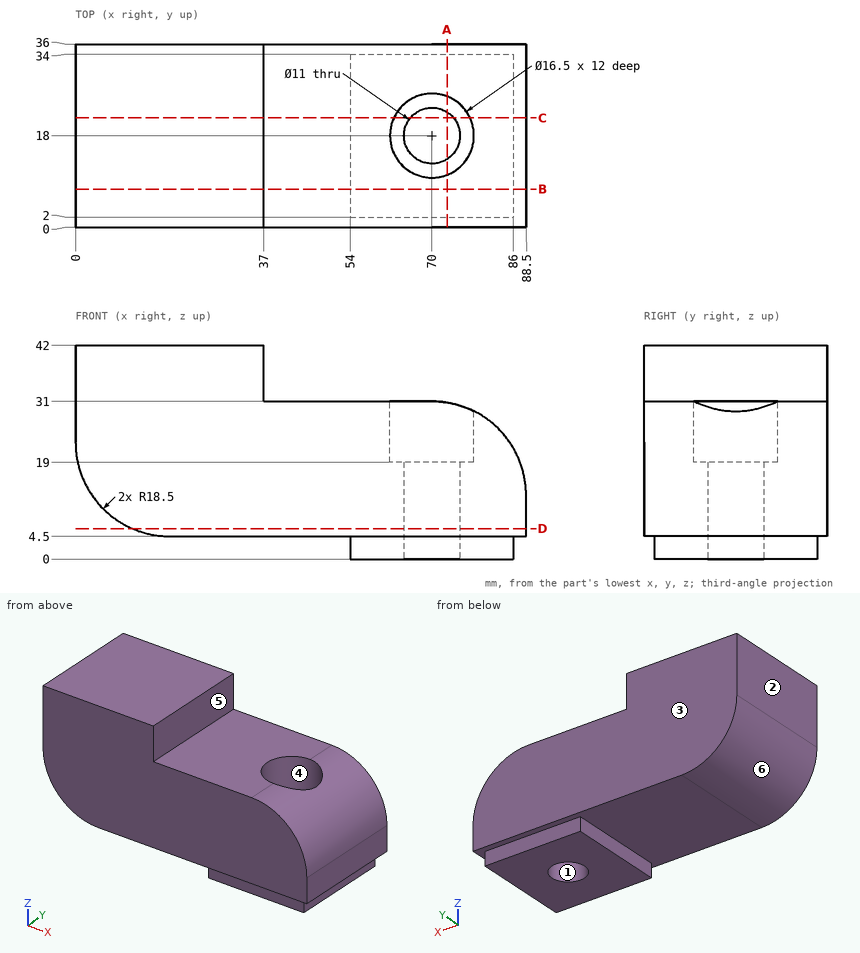
Answer from the drawing. Dimensions are ordinates in mm from the lowest x, y and z of the part. A direction names the side the tool comes from. Round coordinates to 2 decimals unless told otherwise and drop trailing zeros. Write each loop counter-clockwise with the first axis right and the second up, starting at its lowest first coordinate (ties: lowest second). Pieces come first, ordered by that corner, then holes. Notation, with made-up numbers: (59, 41) - (82, 41) arc R27 ccw to (82, 75) - close; hole circle Ø8 at (-3.5, 16). An arc over 180 degrees is marked (long way). One line per item, written item: value.
Q1. Find section A-A (x = 73). Determine the outline of the cut face in (y, z), and give its area (3 significant figures).
The answers:
outline: (0, 4.5) - (2, 4.5) - (2, 0) - (13.39, 0) - (13.39, 19) - (10.31, 19) - (10.31, 30.76) - (0, 30.76) - close; (22.61, 0) - (34, 0) - (34, 4.5) - (36, 4.5) - (36, 30.76) - (25.69, 30.76) - (25.69, 19) - (22.61, 19) - close
area: 733 mm2
Q2. Straight lines are drawn through the part: line 1 (Y direction, x = 70, z = 4); line 2 (Y direction, x = 70, z = 9); line 3 (Z direction, x = 67.5, y = 5.5). For each, find the intervals that lie inside material, in ascending order. Write a range as from..to.
The answers:
line 1: y = 2..12.5, 23.5..34
line 2: y = 0..12.5, 23.5..36
line 3: z = 0..31
Q3. Which of the six approach directions +Z, -Z, +X, -X, +Y, -Y give full straight-line access (tool end or side, diameter ignored) to the marked faces 5 and 6?
The answers:
face 5: +Z, +X, +Y, -Y
face 6: -Z, -X, +Y, -Y
Q4. Find section D-D (z = 6). Determine the outline of the cut face in (x, y).
The answers:
outline: (11.2, 0) - (88.5, 0) - (88.5, 36) - (11.2, 36) - close; hole circle Ø11 at (70, 18)
Q5. Find section B-B (y = 7.5). Determine the outline of the cut face in (x, z), and give its area (3 significant figures).
The answers:
outline: (0, 23) arc R18.5 ccw to (18.5, 4.5) - (54, 4.5) - (54, 0) - (86, 0) - (86, 4.5) - (88.5, 4.5) - (88.5, 12.5) arc R18.5 ccw to (70, 31) - (37, 31) - (37, 42) - (0, 42) - close
area: 2,750 mm2
Q6. Each of these flat-tipped pins is pushed along its axis until it touches: P1, Ø4, axis at y = 29, z = 15, coming from the -X side; P2, Ø5, axis at x = 62.5, z = 1, coming from the +Y side; P3, Ø6.5, axis at x = 70, y = 18, coming from the +Z side; P4, Ø13, axis at x = 66.5, y = 21.5, coming from the +Z side. Where does it stop, or does it pass through?
The answers:
P1: stops at x = 1
P2: stops at y = 34
P3: passes through
P4: stops at z = 31
Q7. For a pull along Y with two mould halves and no side action, classify the marked faces 1, 2, 3 and 4 as pulls with the +Y half, pulls with the -Y half, needs draft (parallel to the pull), parting line crosses it, or undercut.
The answers:
face 1: undercut
face 2: needs draft
face 3: pulls with the +Y half
face 4: undercut
Q8. Find section C-C (y = 21.5). Determine the outline of the cut face in (x, z), and give its area (3 significant figures).
The answers:
outline: (0, 23) arc R18.5 ccw to (18.5, 4.5) - (54, 4.5) - (54, 0) - (65.76, 0) - (65.76, 19) - (62.53, 19) - (62.53, 31) - (37, 31) - (37, 42) - (0, 42) - close; (74.24, 0) - (86, 0) - (86, 4.5) - (88.5, 4.5) - (88.5, 12.5) arc R18.5 ccw to (77.47, 29.42) - (77.47, 19) - (74.24, 19) - close
area: 2,410 mm2
